```python
from build123d import *

# Parameters (mm, degrees)
SKETCH1_R           = 6.35
SKETCH1_R_2         = 11
BOSS_EXTRUDE1_DEPTH = 3
SKETCH3_W           = 515.59682947
SKETCH3_H           = 41.835114591
SKETCH3_H_2         = 39.78804392
CUT_EXTRUDE1_DEPTH  = 4
BOSS_EXTRUDE2_DEPTH = 3
BOSS_EXTRUDE3_DEPTH = 3
FILLET3_R           = 15
SKETCH13_R          = 1.2
SKETCH13_R_2        = 2.25
CUT_EXTRUDE2_DEPTH  = 10
SKETCH14_R          = 1.7
CUT_EXTRUDE3_DEPTH  = 10
BOSS_EXTRUDE5_START = -3
SKETCH16_R          = 6.35
BOSS_EXTRUDE5_DEPTH = 3
SKETCH17_R          = 2.5
CUT_EXTRUDE4_DEPTH  = 10
SKETCH18_R          = 6.35
BOSS_EXTRUDE6_DEPTH = 3
SKETCH19_R          = 3.3
CUT_EXTRUDE5_DEPTH  = 10
SKETCH20_R          = 3.55
CUT_EXTRUDE6_DEPTH  = 50
SKETCH21_R          = 3.5
CUT_EXTRUDE7_DEPTH  = 50
BOSS_EXTRUDE7_START = -3
SKETCH22_R          = 2.5
BOSS_EXTRUDE7_DEPTH = 3
SKETCH23_R          = 3.25
CUT_EXTRUDE8_DEPTH  = 3


with BuildPart() as part:
    # Sketch1 → Boss-Extrude1 (new body)
    with BuildSketch(Plane(origin=(0, 0, 0), x_dir=(1, 0, 0), z_dir=(0, 1, 0))):
        with BuildLine():
            ThreePointArc((-41.906019658, -27.5), (-137.644967441, -71.462113616), (-197, -158.5))
            ThreePointArc((-197, -158.5), (-223.5, -185), (-250, -158.5))
            ThreePointArc((-250, -158.5), (-208.03231281, -72.364423731), (-136.504816256, -8.61145122))
            ThreePointArc((-136.504816256, -8.61145122), (-131.588408281, 0), (-136.504816256, 8.61145122))
            ThreePointArc((-136.504816256, 8.61145122), (-208.03231281, 72.364423731), (-250, 158.5))
            ThreePointArc((-250, 158.5), (-223.5, 185), (-197, 158.5))
            ThreePointArc((-197, 158.5), (-137.644967441, 71.462113616), (-41.906019658, 27.5))
            ThreePointArc((-41.906019658, 27.5), (0, 33.5), (41.906019658, 27.5))
            ThreePointArc((41.906019658, 27.5), (137.644967441, 71.462113616), (197, 158.5))
            ThreePointArc((197, 158.5), (223.5, 185), (250, 158.5))
            ThreePointArc((250, 158.5), (208.03231281, 72.364423731), (136.504816256, 8.61145122))
            ThreePointArc((136.504816256, 8.61145122), (131.588408281, 0), (136.504816256, -8.61145122))
            ThreePointArc((136.504816256, -8.61145122), (208.03231281, -72.364423731), (250, -158.5))
            ThreePointArc((250, -158.5), (223.5, -185), (197, -158.5))
            ThreePointArc((197, -158.5), (137.644967441, -71.462113616), (41.906019658, -27.5))
            ThreePointArc((41.906019658, -27.5), (0, -33.5), (-41.906019658, -27.5))
        make_face()
        with Locations(Location((39.6, 0, 0), (0, 0, 270))):
            Circle(SKETCH1_R, mode=Mode.SUBTRACT)
        with Locations(Location((-39.6, 0, 0), (0, 0, 90))):
            Circle(SKETCH1_R, mode=Mode.SUBTRACT)
        with Locations(Location((0, 0, 0), (0, 0, 270))):
            Circle(SKETCH1_R_2, mode=Mode.SUBTRACT)
    extrude(amount=BOSS_EXTRUDE1_DEPTH)

    # Sketch3 → Cut-Extrude1 (cut)
    with BuildSketch(Plane(origin=(0, 3, 0), x_dir=(1, 0, 0), z_dir=(0, 1, 0))):
        with Locations((7.798414735, 179.417557295)):
            Rectangle(SKETCH3_W, SKETCH3_H)
        with Locations((7.798414735, -178.39402196)):
            Rectangle(SKETCH3_W, SKETCH3_H_2)
    extrude(amount=-CUT_EXTRUDE1_DEPTH, mode=Mode.SUBTRACT)

    # Sketch8 → Boss-Extrude2 (add)
    with BuildSketch(Plane.XZ):
        with BuildLine():
            Line((-250, -158.5), (-250, 158.5))
            ThreePointArc((-250, 158.5), (-223.949910555, 96.121754218), (-182, 43.113663219))
            Line((-182, 43.113663219), (-182, -43.113663219))
            ThreePointArc((-182, -43.113663219), (-223.949910555, -96.121754218), (-250, -158.5))
        make_face()
        with BuildLine():
            Line((-197, -158.5), (-182, -158.5))
            ThreePointArc((-182, -158.5), (-131.938879854, -71.626716928), (-41.906019658, -27.5))
            ThreePointArc((-41.906019658, -27.5), (-137.644967441, -71.462113616), (-197, -158.5))
        make_face()
        with BuildLine():
            Line((250, -158.5), (250, 158.5))
            ThreePointArc((250, 158.5), (223.949910555, 96.121754218), (182, 43.113663219))
            Line((182, 43.113663219), (182, -43.113663219))
            ThreePointArc((182, -43.113663219), (223.949910555, -96.121754218), (250, -158.5))
        make_face()
        with BuildLine():
            Line((-197, 158.5), (-182, 158.5))
            ThreePointArc((-182, 158.5), (-131.938879854, 71.626716928), (-41.906019658, 27.5))
            ThreePointArc((-41.906019658, 27.5), (-137.644967441, 71.462113616), (-197, 158.5))
        make_face()
        with BuildLine():
            Line((197, 158.5), (182, 158.5))
            ThreePointArc((182, 158.5), (131.938879854, 71.626716928), (41.906019658, 27.5))
            ThreePointArc((41.906019658, 27.5), (137.644967441, 71.462113616), (197, 158.5))
        make_face()
        with BuildLine():
            Line((197, -158.5), (182, -158.5))
            ThreePointArc((182, -158.5), (131.938879854, -71.626716928), (41.906019658, -27.5))
            ThreePointArc((41.906019658, -27.5), (137.644967441, -71.462113616), (197, -158.5))
        make_face()
    extrude(amount=-BOSS_EXTRUDE2_DEPTH)

    # Sketch11 → Boss-Extrude3 (add)
    with BuildSketch(Plane(origin=(0, 3, 0), x_dir=(1, 0, 0), z_dir=(0, 1, 0))):
        Polygon((250, 158.5), (250, 173.5), (184.763828731, 173.5), (182, 173.5), (182, 158.5), align=None)
        Polygon((-182, 173.5), (-184.763828731, 173.5), (-250, 173.5), (-250, 158.5), (-182, 158.5), align=None)
    extrude(amount=-BOSS_EXTRUDE3_DEPTH)

    # Fillet3
    fillet3_edges = [part.edges().sort_by_distance(p)[0] for p in [
        (250, 1.5, -173.5),
        (182, 1.5, -173.5),
        (-182, 1.5, -173.5),
        (-250, 1.5, -173.5),
    ]]
    fillet(fillet3_edges, radius=FILLET3_R - 0.0001)  # a hair under: the kernel refuses the full size

    # Sketch13 → Cut-Extrude2 (cut)
    with BuildSketch(Plane(origin=(0, 3, 0), x_dir=(1, 0, 0), z_dir=(0, 1, 0))):
        with Locations(Location((-185.5, -127.333333333, 0), (0, 0, 270))):
            Circle(SKETCH13_R)
        with Locations(Location((-185.5, -103.166666667, 0), (0, 0, 270))):
            Circle(SKETCH13_R)
        with Locations(Location((-246.5, -103.166666667, 0), (0, 0, 270))):
            Circle(SKETCH13_R)
        with Locations(Location((-246.5, -127.333333333, 0), (0, 0, 270))):
            Circle(SKETCH13_R)
        with Locations(Location((-187, -58, 0), (0, 0, 270))):
            Circle(SKETCH13_R_2)
        with Locations(Location((-187, 9, 0), (0, 0, 270))):
            Circle(SKETCH13_R_2)
        with Locations(Location((-187, 76, 0), (0, 0, 270))):
            Circle(SKETCH13_R_2)
        with Locations(Location((-187, 143, 0), (0, 0, 270))):
            Circle(SKETCH13_R_2)
        with Locations(Location((-245, 143, 0), (0, 0, 270))):
            Circle(SKETCH13_R_2)
        with Locations(Location((-245, 76, 0), (0, 0, 270))):
            Circle(SKETCH13_R_2)
        with Locations(Location((-245, 9, 0), (0, 0, 270))):
            Circle(SKETCH13_R_2)
        with Locations(Location((-245, -58, 0), (0, 0, 270))):
            Circle(SKETCH13_R_2)
        with Locations(Location((-242, 163.5, 0), (0, 0, 270))):
            Circle(SKETCH13_R_2)
        with Locations(Location((-190, 163.5, 0), (0, 0, 270))):
            Circle(SKETCH13_R_2)
    cut_extrude2 = extrude(amount=-CUT_EXTRUDE2_DEPTH, mode=Mode.SUBTRACT)

    # Sketch14 → Cut-Extrude3 (cut)
    with BuildSketch(Plane(origin=(0, 3, 0), x_dir=(1, 0, 0), z_dir=(0, 1, 0))):
        with Locations(Location((-194, -146.5, 0), (0, 0, 270))):
            Circle(SKETCH14_R)
        with Locations(Location((-238, -146.5, 0), (0, 0, 270))):
            Circle(SKETCH14_R)
        with Locations(Location((-194, -84.3, 0), (0, 0, 270))):
            Circle(SKETCH14_R)
        with Locations(Location((-238, -84.3, 0), (0, 0, 270))):
            Circle(SKETCH14_R)
    cut_extrude3 = extrude(amount=-CUT_EXTRUDE3_DEPTH, mode=Mode.SUBTRACT)

    # Mirror4: Cut-Extrude2, Cut-Extrude3 across plane
    add(cut_extrude2.mirror(Plane(origin=(0, 0, 0), x_dir=(0, 0, 1), z_dir=(1, 0, 0))), mode=Mode.SUBTRACT)
    add(cut_extrude3.mirror(Plane(origin=(0, 0, 0), x_dir=(0, 0, 1), z_dir=(1, 0, 0))), mode=Mode.SUBTRACT)

    # Sketch16 → Boss-Extrude5 (add)
    with BuildSketch(Plane(origin=(0, 3, 0), x_dir=(1, 0, 0), z_dir=(0, 1, 0)).offset(BOSS_EXTRUDE5_START)):
        with Locations((-39.6, 0)):
            Circle(SKETCH16_R)
        with Locations((39.6, 0)):
            Circle(SKETCH16_R)
    extrude(amount=BOSS_EXTRUDE5_DEPTH)

    # Sketch17 → Cut-Extrude4 (cut)
    with BuildSketch(Plane(origin=(0, 3, 0), x_dir=(1, 0, 0), z_dir=(0, 1, 0))):
        with Locations(Location((0, 19, 0), (0, 0, 270))):
            Circle(SKETCH17_R)
        with Locations(Location((19, 0, 0), (0, 0, 270))):
            Circle(SKETCH17_R)
        with Locations(Location((0, -19, 0), (0, 0, 270))):
            Circle(SKETCH17_R)
        with Locations(Location((-19, 0, 0), (0, 0, 270))):
            Circle(SKETCH17_R)
    extrude(amount=-CUT_EXTRUDE4_DEPTH, mode=Mode.SUBTRACT)

    # Sketch18 → Boss-Extrude6 (add)
    with BuildSketch(Plane.XZ):
        with Locations((-39.6, 0)):
            Circle(SKETCH18_R)
        with Locations((39.6, 0)):
            Circle(SKETCH18_R)
    extrude(amount=-BOSS_EXTRUDE6_DEPTH)

    # Sketch19 → Cut-Extrude5 (cut)
    with BuildSketch(Plane.XZ):
        with Locations(Location((-146.094577254, 48.086735474, 0), (0, 0, 270))):
            Circle(SKETCH19_R)
        with Locations(Location((146.094577254, 48.086735474, 0), (0, 0, 270))):
            Circle(SKETCH19_R)
        with Locations(Location((146.094577254, -48.086735474, 0), (0, 0, 270))):
            Circle(SKETCH19_R)
        with Locations(Location((-146.094577254, -48.086735474, 0), (0, 0, 270))):
            Circle(SKETCH19_R)
    extrude(amount=-CUT_EXTRUDE5_DEPTH, mode=Mode.SUBTRACT)

    # Sketch20 → Cut-Extrude6 (cut)
    with BuildSketch(Plane.XZ):
        with Locations(Location((-239.042094399, -108.501069067, 0), (0, 0, 270))):
            Circle(SKETCH20_R)
        with Locations(Location((-239.042094399, -121.501069067, 0), (0, 0, 270))):
            Circle(SKETCH20_R)
        with Locations(Location((-193.042094399, -108.501069067, 0), (0, 0, 270))):
            Circle(SKETCH20_R)
        with Locations(Location((-193.042094399, -121.501069067, 0), (0, 0, 270))):
            Circle(SKETCH20_R)
    cut_extrude6 = extrude(amount=-CUT_EXTRUDE6_DEPTH, mode=Mode.SUBTRACT)

    # Mirror5: Cut-Extrude6 across plane
    add(cut_extrude6.mirror(Plane(origin=(0, 0, 0), x_dir=(0, 0, 1), z_dir=(1, 0, 0))), mode=Mode.SUBTRACT)

    # Sketch21 → Cut-Extrude7 (cut)
    with BuildSketch(Plane.XZ):
        with Locations(Location((-73.049577254, 0, 0), (0, 0, 270))):
            Circle(SKETCH21_R)
    cut_extrude7 = extrude(amount=-CUT_EXTRUDE7_DEPTH, mode=Mode.SUBTRACT)

    # Mirror6: Cut-Extrude7 across plane
    add(cut_extrude7.mirror(Plane(origin=(0, 0, 0), x_dir=(0, 0, 1), z_dir=(1, 0, 0))), mode=Mode.SUBTRACT)

    # Sketch22 → Boss-Extrude7 (add)
    with BuildSketch(Plane.XZ.offset(BOSS_EXTRUDE7_START)):
        with Locations((0, -19)):
            Circle(SKETCH22_R)
        with Locations((-19, 0)):
            Circle(SKETCH22_R)
        with Locations((0, 19)):
            Circle(SKETCH22_R)
        with Locations((19, 0)):
            Circle(SKETCH22_R)
    extrude(amount=BOSS_EXTRUDE7_DEPTH)

    # Sketch23 → Cut-Extrude8 (cut)
    with BuildSketch(Plane.XZ):
        with Locations(Location((0, 17.25, 0), (0, 0, 270))):
            Circle(SKETCH23_R)
        with Locations(Location((14.938938215, 8.625, 0), (0, 0, 270))):
            Circle(SKETCH23_R)
        with Locations(Location((14.938938215, -8.625, 0), (0, 0, 270))):
            Circle(SKETCH23_R)
        with Locations(Location((0, -17.25, 0), (0, 0, 270))):
            Circle(SKETCH23_R)
        with Locations(Location((-14.938938215, -8.625, 0), (0, 0, 270))):
            Circle(SKETCH23_R)
        with Locations(Location((-14.938938215, 8.625, 0), (0, 0, 270))):
            Circle(SKETCH23_R)
    extrude(amount=-CUT_EXTRUDE8_DEPTH, mode=Mode.SUBTRACT)


solid = part.part
```
Check sheet for the modelled part. Datum: model origin and axes. Units: mm. A direction names the side the tool comes from. Round coordinates to 2 decimals unless told otherwise and drop trailing zeros. Loops run counter-clockwise (first coordinate to the right, second up) from the corner with the lowest first, then second, coordinate; pieces in that order, holes last. Notation, with made-up numbers: (65.5, 33.5) -> (90.5, 33.5) arc R11 cw to (90.5, 37.5) -> close; hole circle Ø5 at (2, -25). An arc over 180 degrees is marked (long way). Answer in a Markdown table with one row per item.
Q1. Set-up check for faces 4 (the face through (-3, 0, 27)), 5 (the face through (186.28, 1.48, -168.99)), 6 (the face through (132.975, 1.479, 72.604)): record each of +Z, -Z, +X, -X, +Y, -Y from which the full face is reachable in a straight line by a thin tool's end or side.
Data:
| item | result |
|---|---|
| face 4 | +Z, -Z, +X, -X, -Y |
| face 5 | -Z, +Y, -Y |
| face 6 | +Z, +Y, -Y |
Q2. Sectioned sample at B-B on y = 1.4. Give the number of separate pieces and of enclosed holes in the cut face, then the cut area to 3 significant figures.
Data:
| item | result |
|---|---|
| separate pieces | 1 |
| enclosed holes | 59 |
| area | 81,000 mm^2 |
Q3. Release check for a two-part mould opening along X. For faces 1 (the face through (159.931, 1.479, 24.305)), 2 (the face through (-3, 3, 32)), 3 (the face through (245.72, 1.48, -168.99)) record: released by +X, released by -X, zero draft, split by the parting line, or undercut.
Data:
| item | result |
|---|---|
| face 1 | undercut |
| face 2 | zero draft |
| face 3 | released by +X |
Q4. Sectioned sample at C-C on x = 60. Enter the section's corners in (y, z).
Data:
| item | result |
|---|---|
| outline | (0, -31.42) -> (3, -31.42) -> (3, 31.42) -> (0, 31.42) -> close |
Q5. Go/stop test with flat-tipped pins: P1, Ø1.5, axis at x = 28.5, y = 2.5, coming from the +Z side; P2, Ø1, axis at x = 120.5, y = 1.5, coming from the -Z side. Record where each tip stops, or that it passes through.
Data:
| item | result |
|---|---|
| P1 | stops at z = 30.9 |
| P2 | stops at z = -62.23 |
Q6. Thickness scan on L1, parallel to X at y = 2.5, z = 2.5; L2, parallel to X at y = 1.4, z = -143; L3, parallel to Z at x = -245, y = 1.25. Record the ranges inside material, lowest first.
Data:
| item | result |
|---|---|
| L1 | x = -250 to -182, -131.91 to -75.5, -70.6 to -10.71, 10.71 to 70.6, 75.5 to 131.91, 182 to 250 |
| L2 | x = -250 to -247.25, -242.75 to -189.25, -184.75 to -177.65, 177.65 to 184.75, 189.25 to 242.75, 247.25 to 250 |
| L3 | z = -169.68 to -145.25, -140.75 to -78.25, -73.75 to -11.25, -6.75 to 55.75, 60.25 to 158.5 |
Q7. Sectioned sample at D-D on x = -121. Enter the section's corners in (y, z).
Data:
| item | result |
|---|---|
| outline | (0, -62.23) -> (3, -62.23) -> (3, 62.23) -> (0, 62.23) -> close |
Q8. Sectioned sample at A-A on x = 166. Enter the section's corners in (y, z), then the cut area to 3 significant figures.
Data:
| item | result |
|---|---|
| outline | (0, -115.92) -> (3, -115.92) -> (3, -29.04) -> (0, -29.04) -> close; (0, 29.04) -> (3, 29.04) -> (3, 115.92) -> (0, 115.92) -> close |
| area | 521 mm^2 |
